from build123d import *

# Parameters (mm, degrees)
F1_DEPTH = 25.4


with BuildPart() as f1:
    # F0 (on Top) → F1 (new body)
    with BuildSketch(Plane.XY):
        with BuildLine():
            ThreePointArc((0, 74.055061), (-74.663883, 0.152692), (0, -73.749676))
            ThreePointArc((0, -73.749676), (74.243208, 0.152692), (0, 74.055061))
        make_face()
        with BuildLine():
            ThreePointArc((-57.023406, -26.218485), (-60.507444, -7.590035), (-60.500612, 11.36142))
            ThreePointArc((-60.500612, 11.36142), (-49.402322, 36.234016), (-30.385477, 55.732161))
            ThreePointArc((-30.385477, 55.732161), (-37.869253, 38.596059), (-39.85231, 20.002501))
            ThreePointArc((-39.85231, 20.002501), (-28.383603, 8.629948), (-12.367958, 6.540619))
            ThreePointArc((-12.367958, 6.540619), (-13.701344, 21.364175), (-12.367958, 36.187731))
            ThreePointArc((-12.367958, 36.187731), (-14.11452, 42.835135), (-12.367958, 49.482539))
            ThreePointArc((-12.367958, 49.482539), (-10.020724, 42.85473), (-7.787234, 36.187731))
            ThreePointArc((-7.787234, 36.187731), (-3.893617, 36.798721), (0, 36.187731))
            ThreePointArc((0, 36.187731), (3.893617, 36.798721), (7.787234, 36.187731))
            ThreePointArc((7.787234, 36.187731), (10.020724, 42.85473), (12.367958, 49.482539))
            ThreePointArc((12.367958, 49.482539), (14.11452, 42.835135), (12.367958, 36.187731))
            ThreePointArc((12.367958, 36.187731), (13.701344, 21.364175), (12.367958, 6.540619))
            ThreePointArc((12.367958, 6.540619), (28.383603, 8.629948), (39.85231, 20.002501))
            ThreePointArc((39.85231, 20.002501), (37.869253, 38.596059), (30.385477, 55.732161))
            ThreePointArc((30.385477, 55.732161), (49.402322, 36.234016), (60.500612, 11.36142))
            ThreePointArc((60.500612, 11.36142), (60.507444, -7.590035), (57.023406, -26.218485))
            ThreePointArc((57.023406, -26.218485), (45.143136, -48.537797), (24.888607, -63.672081))
            ThreePointArc((24.888607, -63.672081), (35.339447, -44.987114), (40.768456, -24.277844))
            ThreePointArc((40.768456, -24.277844), (34.191606, -17.646196), (24.888607, -18.475592))
            ThreePointArc((24.888607, -18.475592), (21.283884, -23.958158), (17.282898, -29.158607))
            ThreePointArc((17.282898, -29.158607), (14.979822, -23.746067), (12.367958, -18.475592))
            ThreePointArc((12.367958, -18.475592), (4.65192, -30.401362), (0, -43.822274))
            ThreePointArc((0, -43.822274), (-4.65192, -30.401362), (-12.367958, -18.475592))
            ThreePointArc((-12.367958, -18.475592), (-14.979822, -23.746067), (-17.282898, -29.158607))
            ThreePointArc((-17.282898, -29.158607), (-21.283884, -23.958158), (-24.888607, -18.475592))
            ThreePointArc((-24.888607, -18.475592), (-34.191606, -17.646196), (-40.768456, -24.277844))
            ThreePointArc((-40.768456, -24.277844), (-35.339447, -44.987114), (-24.888607, -63.672081))
            ThreePointArc((-24.888607, -63.672081), (-45.143136, -48.537797), (-57.023406, -26.218485))
        make_face(mode=Mode.SUBTRACT)
    extrude(amount=F1_DEPTH)


solid = f1.part
Geometry check sheet. Reference: the model listing, model coordinates, mm. Coordinates: 2 decimals unless noted, no trailing zeros. Loops run counter-clockwise (first coordinate to the right, second up) from the corner with the lowest first, then second, coordinate; pieces in that order, holes last. Notation, with made-up numbers: (78, 51) - (117, 51) arc R21 cw to (117, 68) - close; hole circle Ø7 at (64.5, 82.5). An arc over 180 degrees is marked (long way). Use one line per item in the form item = value. Start each with the question number.
Item 1: Section check A-A, the plane x = -9.5. Enter the section's corners in (y, z), and give its area (3 significant figures).
Item 2: Section check B-B, the plane y = -54. Enter the section's corners in (x, z).
Item 3: Section check D-D, the plane y = 39.5. Enter the section's corners in (x, z).
Item 4: Gauge pin test, flat ends, axial feed: pin 1 (6 mm diameter, centred on y = 33, z = 6, fed in from +X); pin 2 (10 mm diameter, centred on x = 34.5, y = 55, fed in from -Z); pin 3 (6 mm diameter, centred on x = -25.5, z = 12.5, fed in from +Y); pin 4 (12 mm diameter, centred on y = -57, z = 13, fed in from -X). Record the tip position at first contact, or that the pin passes through.
Item 5: Thickness scan on probe 1 along X at (y, z) = (-49.5, 15.25); probe 2 along X at (y, z) = (12, 23); probe 3 along X at (y, z) = (-43, 19.75). Record the ranges inside material, lowest first.
Computed:
q1.outline = (-73.23, 0) - (-22.21, 0) - (-22.21, 25.4) - (-73.23, 25.4) - close; (41.33, 0) - (73.54, 0) - (73.54, 25.4) - (41.33, 25.4) - close
q1.area = 2,110 mm2
q2.outline = (-51.05, 0) - (-39.79, 0) - (-39.79, 25.4) - (-51.05, 25.4) - close; (-31.07, 0) - (31.07, 0) - (31.07, 25.4) - (-31.07, 25.4) - close; (39.79, 0) - (50.63, 0) - (50.63, 25.4) - (39.79, 25.4) - close
q3.outline = (-63.32, 0) - (-47.06, 0) - (-47.06, 25.4) - (-63.32, 25.4) - close; (-37.62, 0) - (-13.7, 0) - (-13.7, 25.4) - (-37.62, 25.4) - close; (-8.88, 0) - (8.88, 0) - (8.88, 25.4) - (-8.88, 25.4) - close; (13.7, 0) - (37.62, 0) - (37.62, 25.4) - (13.7, 25.4) - close; (47.06, 0) - (62.9, 0) - (62.9, 25.4) - (47.06, 25.4) - close
q4.pin_1 = 67.95
q4.pin_2 = 0
q4.pin_3 = 70.79
q4.pin_4 = -54.1
q5.probe_1 = -55.5 to -44.3, -33.37 to 33.37, 44.3 to 55.08
q5.probe_2 = -73.71 to -60.34, -33.55 to -13.17, 13.17 to 33.55, 60.34 to 73.29
q5.probe_3 = -60.76 to -49.35, -36.11 to -0.18, 0.18 to 36.11, 49.35 to 60.34
